Could you check a few things on this model? Use its own coordinates, in mm. A direction names the side the tool comes from. Round coordinates to 2 decimals unless told otherwise and drop trailing zeros. Order: outer loops, then holes, each group sorted by start corner. A loop starts at its lowest first (then second) coordinate and runs counter-clockwise, first axis right, second up.
```python
from build123d import *

# Parameters (mm, degrees)
SKETCH006_R     = 29.5
PAD004_DEPTH    = 5
THICKNESS_T     = -2.3
CHAMFER_SIZE    = 1.5
CHAMFER001_SIZE = 0.3


with BuildPart() as part:
    # Sketch006 → Pad004 (new body)
    with BuildSketch(Plane.XY):
        Circle(SKETCH006_R)
    extrude(amount=PAD004_DEPTH)

    # Thickness
    thickness_openings = [part.faces().sort_by_distance(p)[0] for p in [
        (0, 0, 0),
    ]]
    offset(amount=THICKNESS_T, openings=thickness_openings)

    # Chamfer
    chamfer_edges = [part.edges().sort_by_distance(p)[0] for p in [
        (-29.5, 0, 5),
    ]]
    chamfer(chamfer_edges, length=CHAMFER_SIZE)

    # Chamfer001
    chamfer001_edges = [part.edges().sort_by_distance(p)[0] for p in [
        (-28, 0, 5),
    ]]
    chamfer(chamfer001_edges, length=CHAMFER001_SIZE)


with BuildPart() as part_1:
    # Body002 placement: moved
    add(part.part.moved(Location((0, 0, 2))))


solid = part_1.part
```
Q1. I need wall thicknesses on L1, parallel to Y at x = 0, z = 3.95; L2, parallel to Z at x = 6.5, y = 9.5; L3, parallel to X at y = -13.5, z = 4.2. Which ranges of each line are inside material? Lowest first, please.
Q2. We'd pull the mould along X, two halves only. Please class faces 1 (the cylindrical face through (28.14, 8.86, 3.73)), 2 (the cylindrical face through (-5.896, -26.553, 3.331)), 3 (the flat face through (0, 0, 7)): released by +X, released by -X, zero draft, split by the parting line, or undercut.
Q3. For P1, Ø16.5, axis at x = -8, y = 10.5, coming from the -Z side; P2, Ø1.5, axis at y = 2, z = 4.5, coming from the -X side; P3, Ø1.5, axis at x = 8, z = 5, coming from the -Y side, each with a flat end and sliding along its axis, tell me the tip position at first contact or that it passes through.
Q4. For faces 4 (the flat face through (0, 0, 4.7)), 5 (the flat face through (9, -26, 2)), which set-ups out of +Z, -Z, +X, -X, +Y, -Y let a thin tool reach every point of the face, with its end or its side?
Q5. Imagine slicing it at C-C, the plane z = 3.45. Please give me the cut outline in (x, y), then the cut area to 3 significant figures.
Q6. Imagine slicing it at A-A, the plane y = 0. Please give me the cut outline in (x, z).
Filled in:
1. L1: y = -29.5 to -27.2, 27.2 to 29.5
1. L2: z = 4.7 to 7
1. L3: x = -26.23 to -23.61, 23.61 to 26.23
2. face 1: split by the parting line
2. face 2: undercut
2. face 3: zero draft
3. P1: stops at z = 4.7
3. P2: stops at x = -29.47
3. P3: stops at y = -28.6
4. face 4: -Z
4. face 5: -Z, +X, -X, +Y, -Y
5. outline: circle Ø59 at (0, 0); hole circle Ø54.4 at (0, 0)
5. area: 410 mm2
6. outline: (-29.5, 2) - (-27.2, 2) - (-27.2, 4.7) - (27.2, 4.7) - (27.2, 2) - (29.5, 2) - (29.5, 5.5) - (28.21, 6.79) - (27.7, 7) - (-27.7, 7) - (-28.21, 6.79) - (-29.5, 5.5) - close
